from build123d import *

# Parameters (mm, degrees)
SZKIC1_W                            = 70
SZKIC1_H                            = 70
SZKIC1_R                            = 12
DODANIE_WYCI_GNI_CIE1_DEPTH         = 60
SZKIC1_3_R                          = 23.5
WYTNIJ_WYCI_GNI_CIE1_DEPTH          = 3
SZKIC1_4_R                          = 23.5
SZKIC1_4_R_2                        = 20
SZKIC1_4_R_3                        = 12
SZKIC1_4_R_4                        = 16
WYTNIJ_WYCI_GNI_CIE2_DEPTH          = 23
SZKIC1_6_R                          = 16
SZKIC1_6_R_2                        = 12
WYTNIJ_WYCI_GNI_CIE5_DEPTH          = 40
SFAZOWANIE1_SIZE                    = 2
SFAZOWANIE2_SIZE                    = 2
OTW_R_GWINTOWANY_M8X1_01_AT_2_COUNT = 2
OTW_R_GWINTOWANY_M8X1_01_AT_2_PITCH = 50
OTW_R_GWINTOWANY_M8X1_01_AT_3_COUNT = 2
OTW_R_GWINTOWANY_M8X1_01_AT_3_PITCH = 35
OTW_R_GWINTOWANY_M8X1_01_AT_4_COUNT = 2
OTW_R_GWINTOWANY_M8X1_01_AT_4_PITCH = 61.032778079


with BuildPart() as part:
    # Szkic1 → Dodanie-wyci_gni_cie1 (new body)
    with BuildSketch(Plane(origin=(0, 0, 0), x_dir=(1, 0, 0), z_dir=(0, 1, 0))):
        with Locations((35, 35)):
            Rectangle(SZKIC1_W, SZKIC1_H)
        with Locations(Location((35, 35, 0), (0, 0, 270))):
            Circle(SZKIC1_R, mode=Mode.SUBTRACT)
    extrude(amount=DODANIE_WYCI_GNI_CIE1_DEPTH)

    # Szkic1_3 → Wytnij-wyci_gni_cie1 (cut)
    with BuildSketch(Plane(origin=(0, 0, 0), x_dir=(1, 0, 0), z_dir=(0, 1, 0))):
        with BuildLine():
            ThreePointArc((5, 55), (7.928932188, 62.071067812), (15, 65))
            Line((15, 65), (55, 65))
            ThreePointArc((55, 65), (62.071067812, 62.071067812), (65, 55))
            Line((65, 55), (65, 15))
            ThreePointArc((65, 15), (62.071067812, 7.928932188), (55, 5))
            Line((55, 5), (15, 5))
            ThreePointArc((15, 5), (7.928932188, 7.928932188), (5, 15))
            Line((5, 15), (5, 35))
            Line((5, 35), (5, 55))
        make_face()
        with Locations(Location((35, 35, 0), (0, 0, 270))):
            Circle(SZKIC1_3_R, mode=Mode.SUBTRACT)
    extrude(amount=WYTNIJ_WYCI_GNI_CIE1_DEPTH, mode=Mode.SUBTRACT)

    # Szkic1_4 → Wytnij-wyci_gni_cie2 (cut)
    # profile 1 of 4: a face of its own
    with BuildSketch(Plane(origin=(0, 0, 0), x_dir=(1, 0, 0), z_dir=(0, 1, 0))):
        with Locations(Location((35, 35, 0), (0, 0, 270))):
            Circle(SZKIC1_4_R)
        with Locations((35, 35)):
            Circle(SZKIC1_4_R_2, mode=Mode.SUBTRACT)
    # profile 2 of 4: a face of its own
    with BuildSketch(Plane(origin=(0, 0, 0), x_dir=(1, 0, 0), z_dir=(0, 1, 0))):
        with Locations((35, 35)):
            Circle(SZKIC1_4_R_2)
        with Locations(Location((35, 35, 0), (0, 0, 270))):
            Circle(SZKIC1_4_R_3, mode=Mode.SUBTRACT)
    # profile 3 of 4: a face of its own
    with BuildSketch(Plane(origin=(0, 0, 0), x_dir=(1, 0, 0), z_dir=(0, 1, 0))):
        with Locations((35, 35)):
            Circle(SZKIC1_4_R_4)
        with Locations(Location((35, 35, 0), (0, 0, 270))):
            Circle(SZKIC1_4_R_3, mode=Mode.SUBTRACT)
    # profile 4 of 4: a face of its own
    with BuildSketch(Plane(origin=(0, 0, 0), x_dir=(1, 0, 0), z_dir=(0, 1, 0))):
        with Locations(Location((35, 35, 0), (0, 0, 270))):
            Circle(SZKIC1_4_R_3)
    extrude(amount=WYTNIJ_WYCI_GNI_CIE2_DEPTH, mode=Mode.SUBTRACT)

    # Szkic1_6 → Wytnij-wyci_gni_cie5 (cut)
    with BuildSketch(Plane(origin=(0, 0, 0), x_dir=(1, 0, 0), z_dir=(0, 1, 0))):
        with Locations(Location((35, 35, 0), (0, 0, 270))):
            Circle(SZKIC1_6_R)
        with Locations(Location((35, 35, 0), (0, 0, 270))):
            Circle(SZKIC1_6_R_2, mode=Mode.SUBTRACT)
    extrude(amount=WYTNIJ_WYCI_GNI_CIE5_DEPTH, mode=Mode.SUBTRACT)

    # Sfazowanie1
    sfazowanie1_edges = [part.edges().sort_by_distance(p)[0] for p in [
        (35, 40, -47),
    ]]
    chamfer(sfazowanie1_edges, length=SFAZOWANIE1_SIZE)

    # Sfazowanie2
    sfazowanie2_edges = [part.edges().sort_by_distance(p)[0] for p in [
        (35, 3, -58.5),
    ]]
    chamfer(sfazowanie2_edges, length=SFAZOWANIE2_SIZE)

    # Szkic4 → Otw_r gwintowany M8x1.01 (revolve, cut)
    with BuildSketch(Plane(origin=(70, 47.5, -10), x_dir=(0, 0, -1), z_dir=(0, 1, 0))):
        Polygon((0, 0), (0, 10.103012167), (3.5, 8), (3.5, 0), align=None)
    otw_r_gwintowany_m8x1_01 = revolve(axis=Axis((76.35, 47.5, -10), (-1, 0, 0)), mode=Mode.SUBTRACT)

    # Otw_r gwintowany M8x1.01 at 2: Otw_r gwintowany M8x1.01 ×2
    with Locations(*[(0, 0, -i * OTW_R_GWINTOWANY_M8X1_01_AT_2_PITCH) for i in range(1, OTW_R_GWINTOWANY_M8X1_01_AT_2_COUNT)]):
        add(otw_r_gwintowany_m8x1_01, mode=Mode.SUBTRACT)

    # Otw_r gwintowany M8x1.01 at 3: Otw_r gwintowany M8x1.01 ×2
    with Locations(*[(0, -i * OTW_R_GWINTOWANY_M8X1_01_AT_3_PITCH, 0) for i in range(1, OTW_R_GWINTOWANY_M8X1_01_AT_3_COUNT)]):
        add(otw_r_gwintowany_m8x1_01, mode=Mode.SUBTRACT)

    # Otw_r gwintowany M8x1.01 at 4: Otw_r gwintowany M8x1.01 ×2
    with Locations(*[Vector(0, -0.5734623443633283, -0.8192319205190405) * (i * OTW_R_GWINTOWANY_M8X1_01_AT_4_PITCH) for i in range(1, OTW_R_GWINTOWANY_M8X1_01_AT_4_COUNT)]):
        add(otw_r_gwintowany_m8x1_01, mode=Mode.SUBTRACT)

    # Lustro1: Otw_r gwintowany M8x1.01 across plane
    add(otw_r_gwintowany_m8x1_01.mirror(Plane(origin=(35, 0, 0), x_dir=(0, 0, 1), z_dir=(1, 0, 0))), mode=Mode.SUBTRACT)

    # Lustro1 copy 1 sketch → Lustro1 copy 1 (revolve, cut)
    with BuildSketch(Plane(origin=(0, 47.5, -60), x_dir=(0, 0, -1), z_dir=(0, 1, 0))):
        Polygon((0, 0), (0, -10.103012167), (3.5, -8), (3.5, 0), align=None)
    revolve(axis=Axis((-6.35, 47.5, -60), (-1, 0, 0)), mode=Mode.SUBTRACT)

    # Lustro1 copy 2 sketch → Lustro1 copy 2 (revolve, cut)
    with BuildSketch(Plane(origin=(0, 12.5, -10), x_dir=(0, 0, -1), z_dir=(0, 1, 0))):
        Polygon((0, 0), (0, -10.103012167), (3.5, -8), (3.5, 0), align=None)
    revolve(axis=Axis((-6.35, 12.5, -10), (-1, 0, 0)), mode=Mode.SUBTRACT)

    # Lustro1 copy 3 sketch → Lustro1 copy 3 (revolve, cut)
    with BuildSketch(Plane(origin=(0, 12.5, -60), x_dir=(0, 0, -1), z_dir=(0, 1, 0))):
        Polygon((0, 0), (0, -10.103012167), (3.5, -8), (3.5, 0), align=None)
    revolve(axis=Axis((-6.35, 12.5, -60), (-1, 0, 0)), mode=Mode.SUBTRACT)


solid = part.part
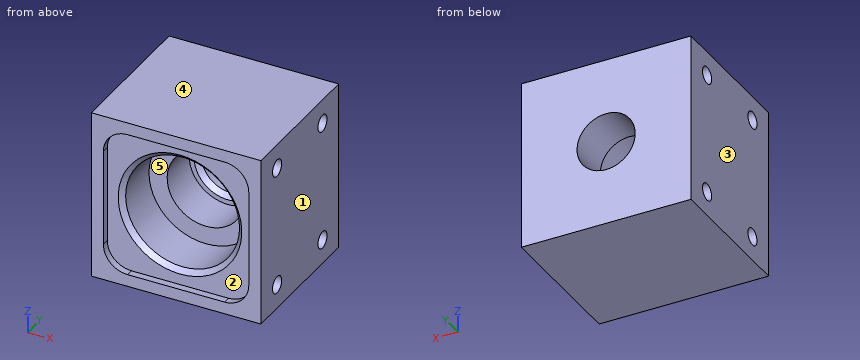
Geometry check sheet. Reference: the model listing, model coordinates, mm. Face numbers are marked on the shaded views. A direction names the side the tool comes from. Coordinates: 2 decimals unless noted, no trailing zeros. Order: outer loops, then holes, each group sorted by start corner. A loop starts at its lowest first (then second) coordinate and runs counter-clockwise, first axis right, second up. Notation, with made-up numbers: M 63,-3.5 L 92,-3.5 A28 ccw 92,15.5 Z; hole C -23,15 d1. An arc over 180 degrees is marked long. Use CSV: the item, a comma, the result in double quotes.
Item 1: Cross-section at D-D on y = 43. Record the cut outline in (x, z).
Returned:
outline,"M 0,-70 L 70,-70 L 70,0 L 0,0 Z; hole C 35,-35 d24"
Item 2: Gauge pin test, flat ends, axial feed: pin 1 Ø12 at (x, z) = (56, -29.5) entering from -Y; pin 2 Ø6.5 at (y, z) = (47.5, -60) entering from -X; pin 3 Ø16 at (x, z) = (37, -28.5) entering from -Y. Record the tip position at first contact, or that the pin passes through.
Returned:
pin 1,"stops at y = 3"
pin 2,"stops at x = 8.15"
pin 3,"stops at y = 40"
Item 3: Cross-section at C-C on y = 7. Record the cut outline in (x, z).
Returned:
outline,"M 0,-70 L 70,-70 L 70,0 L 0,0 Z; hole C 35,-35 d47"
Item 4: Mould release check, pull along X, two halves, no side actions. Record for the marked faces 1, 2 and 3: pulls with the +X half, pulls with the -X half, needs draft (parallel to the pull), parting line crosses it, or undercut.
Returned:
face 1,"pulls with the +X half"
face 2,"undercut"
face 3,"pulls with the -X half"
Item 5: Tool access check on the marked faces 4 and 5. Record the directions out of +Z, -Z, +X, -X, +Y, -Y that give a thin tool (end or side, any length) a straight path to the whole face; none if there is none.
Returned:
face 4,"+Z, +X, -X, +Y, -Y"
face 5,"-Y"
Item 6: Cross-section at A-A on z = -35. Record the cut outline in (x, y).
Returned:
outline,"M 0,0 L 5,0 L 5,3 L 9.5,3 L 11.5,5 L 11.5,23 L 19,23 L 19,40 L 21,40 L 23,42 L 23,60 L 0,60 Z; M 47,42 L 49,40 L 51,40 L 51,23 L 58.5,23 L 58.5,5 L 60.5,3 L 65,3 L 65,0 L 70,0 L 70,60 L 47,60 Z"
Item 7: Cross-section at B-B on x = 35. Record the cut outline in (y, z), then the cut area to 3 significant figures.
Returned:
outline,"M 0,-70 L 60,-70 L 60,-47 L 42,-47 L 40,-49 L 40,-51 L 23,-51 L 23,-58.5 L 5,-58.5 L 3,-60.5 L 3,-65 L 0,-65 Z; M 0,-5 L 3,-5 L 3,-9.5 L 5,-11.5 L 23,-11.5 L 23,-19 L 40,-19 L 40,-21 L 42,-23 L 60,-23 L 60,0 L 0,0 Z"
area,"2,050 mm2"
Item 8: Thickness scan on line 1 along Z through (x, y) = (2.25, 12.5); line 2 along Y through (x, z) = (67, -60); line 3 along X through (y, z) = (47, -35.5). Record the ranges inside material, lowest first.
Returned:
line 1,"z = -70 to -63.5, -56.5 to -13.5, -6.5 to 0"
line 2,"y = 0 to 9, 16 to 44, 51 to 60"
line 3,"x = 0 to 23.01, 46.99 to 70"
